Design review of the part built by this model. Coordinates are the model's own, in mm. A direction names the side the tool comes from. Round coordinates to 2 decimals unless told otherwise and drop trailing zeros. Loops run counter-clockwise (first coordinate to the right, second up) from the corner with the lowest first, then second, coordinate; pieces in that order, holes last. Notation, with made-up numbers: M 57.5,-9.5 L 62.5,-9.5 A31 ccw 62.5,16.5 Z; hole C 87,38.25 d7. An arc over 180 degrees is marked long. Use a Markdown table: item, result.
from build123d import *

# Parameters (mm, degrees)
SKETCH_1_R          = 2
EXTRUDE_1_DEPTH     = 3.8
SKETCH_2_R          = 1.65
EXTRUDE_2_DEPTH     = 1.4
CUT_EXTRUDE_1_DEPTH = 20.207810911
CUT_EXTRUDE_2_DEPTH = 13.660568708


with BuildPart() as part:
    # 草图1 → 凸台-拉伸1 (new body)
    with BuildSketch(Plane(origin=(0, 0, 0), x_dir=(1, 0, 0), z_dir=(0, 1, 0))):
        with Locations(Location((0, 0, 0), (0, 0, 90))):
            Circle(SKETCH_1_R)
    extrude(amount=EXTRUDE_1_DEPTH)

    # 草图2 → 凸台-拉伸2 (add)
    with BuildSketch(Plane(origin=(0, 3.8, 0), x_dir=(1, 0, 0), z_dir=(0, 1, 0))):
        with BuildLine():
            Line((-3.5, 0), (-3.5, 15))
            ThreePointArc((-3.5, 15), (0, 18.5), (3.5, 15))
            Line((3.5, 15), (3.5, 0))
            ThreePointArc((3.5, 0), (0, -3.5), (-3.5, 0))
        make_face()
        with Locations(Location((0, 15, 0), (0, 0, 270))):
            Circle(SKETCH_2_R, mode=Mode.SUBTRACT)
    extrude(amount=EXTRUDE_2_DEPTH)

    # 草图3 → 切除-拉伸1 (cut, through all)
    with BuildSketch(Plane.XZ.offset(-3.8)):
        with BuildLine():
            Line((0, 3.5), (0, 2))
            ThreePointArc((0, 2), (2, 0), (0, -2))
            Line((0, -2), (0, -7.5))
            Line((0, -7.5), (3.5, -7.5))
            Line((3.5, -7.5), (3.5, 0))
            ThreePointArc((3.5, 0), (2.474873734, 2.474873734), (0, 3.5))
        make_face()
    extrude(amount=-CUT_EXTRUDE_1_DEPTH, mode=Mode.SUBTRACT)

    # 草图4 → 切除-拉伸2 (cut, through all)
    with BuildSketch(Plane.XY.offset(-7.5)):
        Polygon((0, 5.2), (3.5, 3.8), (3.5, 5.2), align=None)
    extrude(amount=CUT_EXTRUDE_2_DEPTH, mode=Mode.SUBTRACT)


solid = part.part
1. Take a section at B-B on z = -1.25. Give the boundary of the cut face in (x, y).
Check values:
| item | result |
|---|---|
| outline | M -3.5,3.8 L -1.56,3.8 L -1.56,0 L 1.56,0 L 1.56,4.58 L 0,5.2 L -3.5,5.2 Z |
2. Take a section at A-A on y = 4. Give the boundary of the cut face in (x, z), and give its area (3 significant figures).
Check values:
| item | result |
|---|---|
| outline | M -3.5,-15 A3.5 ccw 3.5,-15 L 3.5,-7.5 L 0,-7.5 L 0,-2 A2 ccw 0,2 L 0,3.5 A3.5 ccw -3.5,0 Z; hole C 0,-15 d3.3 |
| area | 105 mm² |
3. Wall thickness on line 1 along X through (y, z) = (4.25, -15); line 2 along X through (y, z) = (4.35, -14.25); line 3 along Y through (x, z) = (1.25, -8.75): over which ranges is each line inside the solid? List them lowest first. Write a range as from..to.
Check values:
| item | result |
|---|---|
| line 1 | x = -3.5..-1.65, 1.65..3.5 |
| line 2 | x = -3.5..-1.47, 1.47..3.5 |
| line 3 | y = 3.8..5.2 |
4. Take a section at C-C on y = 0.75. Give the boundary of the cut face in (x, z), and give its area (3 significant figures).
Check values:
| item | result |
|---|---|
| outline | C 0,0 d4 |
| area | 12.6 mm² |
5. Machinability: for faces 1 (the face through (0.764, 4.894, -0.028)), 2 (the face through (0, 4, 3)), 3 (the face through (3.5, 4, -11)), which of the approach directions +Z, -Z, +X, -X, +Y, -Y give a long, thin tool a straight path to every point of the face, cutting with its end or side? Answer none if there is none.
Check values:
| item | result |
|---|---|
| face 1 | +Z, +X, +Y |
| face 2 | +Z, +X, +Y, -Y |
| face 3 | +Z, -Z, +X, +Y, -Y |
6. Take a section at D-D on x = -3. Give the boundary of the cut face in (y, z), and give its area (3 significant figures).
Check values:
| item | result |
|---|---|
| outline | M 3.8,-16.8 L 5.2,-16.8 L 5.2,1.8 L 3.8,1.8 Z |
| area | 26.0 mm² |
7. Insertion check: pin 1 (1.1 mm diameter, centred on y = 4.5, z = -4.5, fed in from +X); pin 2 (1.5 mm diameter, centred on x = -1.5, y = 3.5, fed in from -Z); pin 3 (1 mm diameter, centred on x = 1.5, y = 1.5, fed in from +Z); pin 4 (1 mm diameter, centred on y = 2.5, z = -8, fed in from -X). Each pin has a flat end and moves straight along its axis. Give the tip position at first contact, or say it passes through.
Check values:
| item | result |
|---|---|
| pin 1 | stops at x = 0 |
| pin 2 | stops at z = -18.4 |
| pin 3 | stops at z = 1.73 |
| pin 4 | passes through |
8. The part is to be moulded in two halves that separate along X. For faces 4 (the face through (-2.45, 4.49, 2.5)), 5 (the face through (-0.632, 4.49, -13.476)), 6 (the face through (0, 0, 0)), 7 (the face through (0, 4, -5)), say which applies: pulls with the +X half, pulls with the -X half, needs draft (parallel to the pull), parting line crosses it, or undercut.
Check values:
| item | result |
|---|---|
| face 4 | pulls with the -X half |
| face 5 | undercut |
| face 6 | needs draft |
| face 7 | pulls with the +X half |
